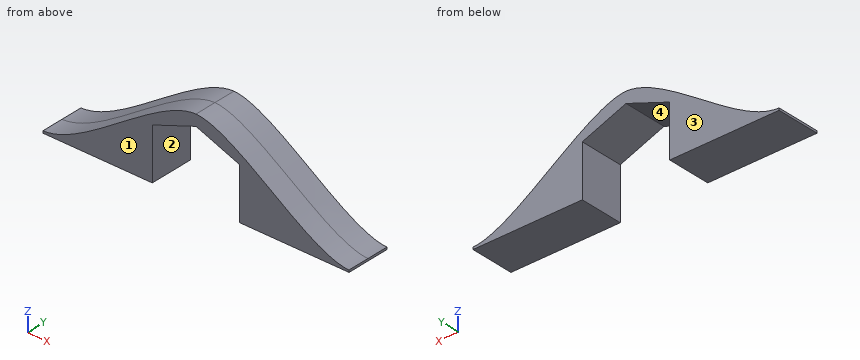
from build123d import *

# Parameters (mm, degrees)
F1_DEPTH = 12.7
F2_W     = 63.5
F2_H     = 25.4
F3_DEPTH = 1.27


with BuildPart() as f1:
    # F0 (on Front) → F1 (new body, symmetric)
    with BuildSketch(Plane.XZ):
        with BuildLine():
            Line((25.4, 28.575), (25.4, 0))
            Line((25.4, 0), (88.9, 0))
            add(Edge.make_bspline(
                [(0, 44.45), (23.8007288426, 43.8667871058), (65.3088388513, 0), (88.9, 0)],
                knots=[0, 0, 0, 0, 99.3932215999, 99.3932215999, 99.3932215999, 99.3932215999], degree=3))
            Line((0, 44.45), (0, 38.1))
            Line((0, 38.1), (25.4, 28.575))
        make_face()
    extrude(amount=F1_DEPTH, both=True)

    # F2 (on face) → F3 (join)
    with BuildSketch(Plane(origin=(0, 0, 0), x_dir=(1, 0, 0), z_dir=(0, 0, -1))):
        with Locations((57.15, 0)):
            Rectangle(F2_W, F2_H)
    extrude(amount=F3_DEPTH)

    # F4: F1 across face


with BuildPart() as f1_1:
    add(f1.part)
    add(f1.part.mirror(Plane(origin=(0, 0, 41.275), x_dir=(0, -1, 0), z_dir=(-1, 0, 0))))


solid = f1_1.part
Geometry check sheet. Reference: the model listing, model coordinates, mm. Face numbers are marked on the shaded views. A direction names the side the tool comes from. Coordinates: 2 decimals unless noted, no trailing zeros. One line per question, with ' | ' between items.
1. Draft check along X on the marked faces 1 and 2. Enter one of: +X half, -X half, draft (parallel to the pull), parting line (faces both ways), or undercut.
Answers:
face 1: draft | face 2: undercut
2. Set-up check for the marked faces 3 and 4: record each of +Z, -Z, +X, -X, +Y, -Y from which the full face is reachable in a straight line by a thin tool's end or side.
Answers:
face 3: +Z, -Z, +X, -X, +Y | face 4: -Z, +Y, -Y
3. Thickness scan on probe 1 along X at (y, z) = (-6.25, 11.5); probe 2 along X at (y, z) = (2.25, 19); probe 3 along Z at (x, y) = (-71, -1.5). Record the ranges inside material, lowest first. Write a range as from..to.
Answers:
probe 1: x = -60.49..-25.4, 25.4..60.49 | probe 2: x = -48.98..-25.4, 25.4..48.98 | probe 3: z = -1.27..5.5
4. Depth check by flat-ended pin: pin 1 Ø1.5 at (y, z) = (-4, 19.5) entering from -X; pin 2 Ø5 at (y, z) = (0.5, 8.5) entering from -X; pin 3 Ø8 at (x, y) = (51.5, -3) entering from +Z. Enter the tip coordinate at first touch or a pass-through.
Answers:
pin 1: stops at x = -49.35 | pin 2: stops at x = -70.02 | pin 3: stops at z = 20
